```python
from build123d import *

# Parameters (mm, degrees)
SKETCH2_W           = 34
SKETCH2_H           = 34
BOSS_EXTRUDE2_DEPTH = 1
FILLET1_R           = 2
SKETCH3_W           = 13.5
SKETCH3_H           = 13.5
BOSS_EXTRUDE3_DEPTH = 6
SKETCH4_R           = 6
BOSS_EXTRUDE4_DEPTH = 5
FILLET2_R           = 0.5
SKETCH5_R           = 5.5
BOSS_EXTRUDE5_DEPTH = 6
SKETCH6_R           = 6
SKETCH6_R_2         = 3
BOSS_EXTRUDE6_DEPTH = 3
SKETCH7_R           = 1
SKETCH7_R_2         = 1.25
CUT_EXTRUDE1_DEPTH  = 32.272991542
FILLET3_R           = 0.5


with BuildPart() as part:
    # Sketch2 → Boss-Extrude2 (new body)
    with BuildSketch(Plane(origin=(0, 0, 0), x_dir=(1, 0, 0), z_dir=(0, 1, 0))):
        Rectangle(SKETCH2_W, SKETCH2_H)
    extrude(amount=BOSS_EXTRUDE2_DEPTH)

    # Fillet1
    fillet1_edges = [part.edges().sort_by_distance(p)[0] for p in [
        (17, 0.5, 17),
        (-17, 0.5, 17),
        (-17, 0.5, -17),
        (17, 0.5, -17),
    ]]
    fillet(fillet1_edges, radius=FILLET1_R)

    # Sketch3 → Boss-Extrude3 (add)
    with BuildSketch(Plane(origin=(0, 1, 0), x_dir=(1, 0, 0), z_dir=(0, 1, 0))):
        Rectangle(SKETCH3_W, SKETCH3_H)
    extrude(amount=BOSS_EXTRUDE3_DEPTH)

    # Sketch4 → Boss-Extrude4 (add)
    with BuildSketch(Plane(origin=(0, 7, 0), x_dir=(1, 0, 0), z_dir=(0, 1, 0))):
        with Locations(Location((0, 0, 0), (0, 0, 270))):
            Circle(SKETCH4_R)
    extrude(amount=BOSS_EXTRUDE4_DEPTH)

    # Fillet2
    fillet2_edges = [part.edges().sort_by_distance(p)[0] for p in [
        (6.75, 4, 6.75),
        (6.75, 4, -6.75),
        (-6.75, 4, -6.75),
        (-6.75, 4, 6.75),
        (6.75, 7, 0),
        (0, 7, -6.75),
        (-6.75, 7, 0),
        (0, 7, 6.75),
    ]]
    fillet(fillet2_edges, radius=FILLET2_R)

    # Sketch5 → Boss-Extrude5 (add)
    with BuildSketch(Plane(origin=(0, 12, 0), x_dir=(1, 0, 0), z_dir=(0, 1, 0))):
        with Locations(Location((0, 0, 0), (0, 0, 270))):
            Circle(SKETCH5_R)
    extrude(amount=BOSS_EXTRUDE5_DEPTH)

    # Sketch6 → Boss-Extrude6 (add)
    with BuildSketch(Plane(origin=(0, 18, 0), x_dir=(1, 0, 0), z_dir=(0, 1, 0))):
        with Locations(Location((0, 0, 0), (0, 0, 270))):
            Circle(SKETCH6_R)
        with Locations(Location((0, 0, 0), (0, 0, 270))):
            Circle(SKETCH6_R_2, mode=Mode.SUBTRACT)
    extrude(amount=BOSS_EXTRUDE6_DEPTH)

    # Sketch7 → Cut-Extrude1 (cut, through all)
    with BuildSketch(Plane(origin=(0, 1, 0), x_dir=(1, 0, 0), z_dir=(0, 1, 0))):
        with Locations((-15.414213562, -15.414213562)):
            Circle(SKETCH7_R)
        with Locations((-14, -14)):
            Circle(SKETCH7_R_2)
        with Locations((15.414213562, -15.414213562)):
            Circle(SKETCH7_R)
        with Locations((14, -14)):
            Circle(SKETCH7_R_2)
        with Locations((15.414213562, 15.414213562)):
            Circle(SKETCH7_R)
        with Locations((14, 14)):
            Circle(SKETCH7_R_2)
        with Locations((-15.414213562, 15.414213562)):
            Circle(SKETCH7_R)
        with Locations((-14, 14)):
            Circle(SKETCH7_R_2)
    extrude(amount=-CUT_EXTRUDE1_DEPTH, mode=Mode.SUBTRACT)

    # Fillet3
    fillet3_edges = [part.edges().sort_by_distance(p)[0] for p in [
        (-14.444967533, 0.5, -15.168119812),
        (-15.168119812, 0.5, -14.444967533),
        (15.168119812, 0.5, -14.444967533),
        (14.444967533, 0.5, -15.168119812),
        (14.444967533, 0.5, 15.168119812),
        (15.168119812, 0.5, 14.444967533),
        (-15.168119812, 0.5, 14.444967533),
        (-14.444967533, 0.5, 15.168119812),
    ]]
    fillet(fillet3_edges, radius=FILLET3_R)


solid = part.part
```
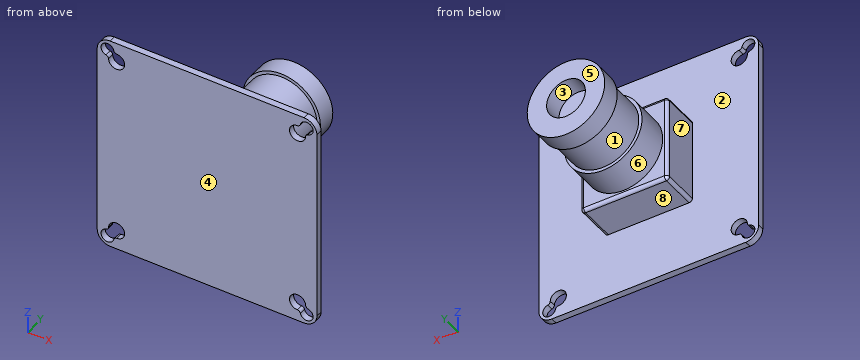
Build history of the part. All positions in model axes, mm. Face numbers are marked on the shaded views. A direction names the side the tool comes from. Coordinates: 2 decimals unless noted, no trailing zeros. Order: outer loops, then holes, each group sorted by start corner. A loop starts at its lowest first (then second) coordinate and runs counter-clockwise, first axis right, second up. Notation, with made-up numbers: M 38.25,39.5 L 68.25,39.5 A9 ccw 68.25,56.5 Z; hole C -25,11 d4. An arc over 180 degrees is marked long. One line per question, with ' | ' between items. Start each with the question number.
1. Mould opens along Y. For the marked faces 1, 2, 3 and 4 say: +Y half, -Y half, draft (parallel to the pull), parting line (faces both ways), or undercut.
2. Wall check: line 1 along Z through (x, y) = (-14, 0.6); line 2 along Y through (x, z) = (13, 10). Give the ranges that are in metal, low to high. Write a range as [from, to].
3. Flat gauge pins, fed straight in: P1, Ø1.5, axis at x = 14, z = -14, coming from the -Y side; P2, Ø2.5, axis at x = -15.41, z = 15.41, coming from the +Y side; P3, Ø12, axis at x = 6, y = 9, coming from the +Z side; P4, Ø10, axis at x = -3, y = 14, coming from the -Z side. Where does each tip first touch, or does it go through?
4. Cut at B-B (z = 0). Write the cut outline in (x, y).
5. Cut at A-A (x = 0). Write the cut outline in (y, z).
6. Cut at C-C (y = 8.25). Write the cut outline in (x, z), plus the area to 3 significant figures.
7. Tool access for the marked faces 5, 6, 7 and 8: list every direction of +Z, -Z, +X, -X, +Y, -Y with a clear straight run to the whole face (end or side of a thin tool).
8. Cut at D-D (z = -10). Write the cut outline in (x, y).
The answers:
1) face 1: undercut | face 2: +Y half | face 3: draft | face 4: -Y half
2) line 1: z = [-17, -15.25], [-12.75, 12.75], [15.25, 17] | line 2: y = [0, 1]
3) P1: passes through | P2: stops at y = 1 | P3: stops at z = 6.75 | P4: stops at z = -6
4) outline: M -17,0 L 17,0 L 17,1 L 6.75,1 L 6.75,6.5 A0.5 ccw 6.25,7 L 6,7 L 6,12 L 5.5,12 L 5.5,18 L 6,18 L 6,21 L 3,21 L 3,18 L -3,18 L -3,21 L -6,21 L -6,18 L -5.5,18 L -5.5,12 L -6,12 L -6,7 L -6.25,7 A0.5 ccw -6.75,6.5 L -6.75,1 L -17,1 Z
5) outline: M 0,-17 L 1,-17 L 1,-6.75 L 6.5,-6.75 A0.5 ccw 7,-6.25 L 7,-6 L 12,-6 L 12,-5.5 L 18,-5.5 L 18,-6 L 21,-6 L 21,-3 L 18,-3 L 18,3 L 21,3 L 21,6 L 18,6 L 18,5.5 L 12,5.5 L 12,6 L 7,6 L 7,6.25 A0.5 ccw 6.5,6.75 L 1,6.75 L 1,17 L 0,17 Z
6) outline: C 0,0 d12 | area: 113 mm2
7) face 5: +Z, -Z, +X, -X, +Y | face 6: +Y | face 7: +Z, -Z, -X, +Y | face 8: -Z, +X, -X, +Y
8) outline: M -17,0 L 17,0 L 17,1 L -17,1 Z
